The model under review builds one solid part; all positions refer to its coordinate system, in mm. A direction names the side the tool comes from. Round coordinates to 2 decimals unless told otherwise and drop trailing zeros. Write each loop counter-clockwise with the first axis right and the second up, starting at its lowest first coordinate (ties: lowest second). Pieces come first, ordered by that corner, then holes. Notation, with made-up numbers: M 3,-37.75 L 43,-37.75 A20 ccw 43,-30.75 Z; hole C -24,-23 d9. An arc over 180 degrees is marked long. One line per item, written item: value. Start each with the question number.
1) Wall thickness on probe 1 along Y at (x, z) = (16.5, -10.5); probe 2 along X at (y, z) = (-7, -17.5); probe 3 along X at (y, z) = (-14, 0.5): over which ranges is each line inside the solid? List them lowest first.
2) Tool access review of faces 1 (the face through (-3.78, 25.2, 2.9)), 2 (the face through (-3.78, -17.37, 2.9)), 3 (the face through (-5.506, 0.156, 24.796)): name each direction out of +Z, -Z, +X, -X, +Y, -Y from which nothing blocks a thin tool from reaching the whole face with its end or side.
3) Take a section at B-B, the plane z = 0. Write out the cut boundary in (x, y), and give its area (3 significant figures).
4) For P1, Ø10, axis at y = 1, z = 13, coming from the +X side; P2, Ø6, axis at x = -12.5, z = 19, coming from the +Y side; P3, Ø2, axis at y = 6.5, z = 13, coming from the -X side; P4, Ø10, axis at y = -16.5, z = 13.5, coming from the -X side, all flat-tipped, find the tip position at first contact; note any pin that passes through.
5) Take a section at A-A, the plane x = 0. Write out the cut boundary in (y, z).
6) Take a section at C-C, the plane y = -2. Write out the cut boundary in (x, z).
7) Take a section at D-D, the plane y = -13. Write out the cut boundary in (x, z) (1 decimal).
from build123d import *

# Parameters (mm, degrees)
SKETCH1_R           = 25.4
BOSS_EXTRUDE1_DEPTH = 11.1125
SKETCH2_R           = 4.7625
BOSS_EXTRUDE2_DEPTH = 28.575
SKETCH3_R           = 4.7625
CUT_EXTRUDE1_DEPTH  = 15.875


with BuildPart() as part:
    # Sketch1 → Boss-Extrude1 (new body, symmetric)
    with BuildSketch(Plane(origin=(0, 0, 0), x_dir=(1, 0, 0), z_dir=(0, 1, 0))):
        Circle(SKETCH1_R)
    extrude(amount=BOSS_EXTRUDE1_DEPTH, both=True)

    # Sketch2 → Boss-Extrude2 (add)
    with BuildSketch(Plane(origin=(0, 11.1125, 0), x_dir=(1, 0, 0), z_dir=(0, 1, 0))):
        Circle(SKETCH2_R)
    boss_extrude2 = extrude(amount=BOSS_EXTRUDE2_DEPTH)

    # Mirror1: Boss-Extrude2 across plane
    add(boss_extrude2.mirror(Plane.ZX))

    # Sketch3 → Cut-Extrude1 (cut)
    with BuildSketch(Plane(origin=(0, -39.6875, 0), x_dir=(-1, 0, 0), z_dir=(0, -1, 0))):
        Circle(SKETCH3_R)
    extrude(amount=-CUT_EXTRUDE1_DEPTH, mode=Mode.SUBTRACT)


solid = part.part
Checked values:
1. probe 1: y = -11.11 to 11.11
1. probe 2: x = -18.41 to 18.41
1. probe 3: x = -4.74 to 4.74
2. face 1: +Y
2. face 2: -Y
2. face 3: +Y, -Y
3. outline: M -25.4,-11.11 L -4.76,-11.11 L -4.76,-23.81 L 4.76,-23.81 L 4.76,-11.11 L 25.4,-11.11 L 25.4,11.11 L 4.76,11.11 L 4.76,39.69 L -4.76,39.69 L -4.76,11.11 L -25.4,11.11 Z
3. area: 1,520 mm2
4. P1: stops at x = 24.11
4. P2: stops at y = 11.11
4. P3: stops at x = -22.39
4. P4: passes through
5. outline: M -23.81,-4.76 L -11.11,-4.76 L -11.11,-25.4 L 11.11,-25.4 L 11.11,-4.76 L 39.69,-4.76 L 39.69,4.76 L 11.11,4.76 L 11.11,25.4 L -11.11,25.4 L -11.11,4.76 L -23.81,4.76 Z
6. outline: C 0,0 d50.8
7. outline: C 0,0 d9.5
